```python
from build123d import *

# Parameters (mm, degrees)
CYLINDER003_R     = 3.4
CYLINDER003_DEPTH = 10
CYLINDER004_R     = 1.7
CYLINDER004_DEPTH = 9.6
CYLINDER002_R     = 3.4
CYLINDER002_DEPTH = 10
CYLINDER001_R     = 1.7
CYLINDER001_DEPTH = 9.6
CYLINDER008_R     = 3.4
CYLINDER008_DEPTH = 10
CYLINDER006_R     = 1.7
CYLINDER006_DEPTH = 9.6
CYLINDER005_R     = 3.4
CYLINDER005_DEPTH = 10
CYLINDER007_R     = 1.7
CYLINDER007_DEPTH = 9.6
PAD002_DEPTH      = 2
BOX001_W          = 53
BOX001_H          = 62
BOX001_DEPTH      = 2
FILLET_R          = 3
SKETCH001_W       = 21
SKETCH001_H       = 32
PAD001_DEPTH      = 2


with BuildPart() as grab_screw_head001:
    # Cone002 → Cone002 (revolve)
    with BuildSketch(Plane.XZ):
        Polygon((0, 0), (1.7, 0), (3.4, 3.4), (0, 3.4), align=None)
    revolve(axis=Axis((0, 0, 0), (0, 0, 1)))


with BuildPart() as grab_screw_head_extension001:
    # Cylinder003 → Cylinder003 (new body)
    with BuildSketch(Plane.XY.offset(3.4)):
        Circle(CYLINDER003_R)
    extrude(amount=CYLINDER003_DEPTH)


with BuildPart() as grab_screw001:
    # Cylinder004 → Cylinder004 (new body)
    with BuildSketch(Plane.XY.offset(-9.6)):
        Circle(CYLINDER004_R)
    extrude(amount=CYLINDER004_DEPTH)

    # Fusion002: union grab-screw-head001, grab-screw-head-extension001
    add(grab_screw_head001.part)
    add(grab_screw_head_extension001.part)


with BuildPart() as grab_screw001_1:
    # Fusion002 placement: moved
    add(grab_screw001.part.moved(Location((42, 56, 5))))


with BuildPart() as grab_screw_head:
    # Cone001 → Cone001 (revolve)
    with BuildSketch(Plane.XZ):
        Polygon((0, 0), (1.7, 0), (3.4, 3.4), (0, 3.4), align=None)
    revolve(axis=Axis((0, 0, 0), (0, 0, 1)))


with BuildPart() as grab_screw_head_extension:
    # Cylinder002 → Cylinder002 (new body)
    with BuildSketch(Plane.XY.offset(3.4)):
        Circle(CYLINDER002_R)
    extrude(amount=CYLINDER002_DEPTH)


with BuildPart() as right_screws:
    # Cylinder001 → Cylinder001 (new body)
    with BuildSketch(Plane.XY.offset(-9.6)):
        Circle(CYLINDER001_R)
    extrude(amount=CYLINDER001_DEPTH)

    # Fusion001: union grab-screw-head, grab-screw-head-extension
    add(grab_screw_head.part)
    add(grab_screw_head_extension.part)


with BuildPart() as right_screws_1:
    # Fusion001 placement: moved
    add(right_screws.part.moved(Location((42, 0, 5))))

    # Fusion: union grab-screw001
    add(grab_screw001_1.part)


with BuildPart() as grab_screw_head003:
    # Cone004 → Cone004 (revolve)
    with BuildSketch(Plane.XZ):
        Polygon((0, 0), (1.7, 0), (3.4, 3.4), (0, 3.4), align=None)
    revolve(axis=Axis((0, 0, 0), (0, 0, 1)))


with BuildPart() as grab_screw_head_extension003:
    # Cylinder008 → Cylinder008 (new body)
    with BuildSketch(Plane.XY.offset(3.4)):
        Circle(CYLINDER008_R)
    extrude(amount=CYLINDER008_DEPTH)


with BuildPart() as grab_screw002:
    # Cylinder006 → Cylinder006 (new body)
    with BuildSketch(Plane.XY.offset(-9.6)):
        Circle(CYLINDER006_R)
    extrude(amount=CYLINDER006_DEPTH)

    # Fusion004: union grab-screw-head003, grab-screw-head-extension003
    add(grab_screw_head003.part)
    add(grab_screw_head_extension003.part)


with BuildPart() as grab_screw002_1:
    # Fusion004 placement: moved
    add(grab_screw002.part.moved(Location((42, 56, 5))))


with BuildPart() as grab_screw_head002:
    # Cone003 → Cone003 (revolve)
    with BuildSketch(Plane.XZ):
        Polygon((0, 0), (1.7, 0), (3.4, 3.4), (0, 3.4), align=None)
    revolve(axis=Axis((0, 0, 0), (0, 0, 1)))


with BuildPart() as grab_screw_head_extension002:
    # Cylinder005 → Cylinder005 (new body)
    with BuildSketch(Plane.XY.offset(3.4)):
        Circle(CYLINDER005_R)
    extrude(amount=CYLINDER005_DEPTH)


with BuildPart() as all_screws:
    # Cylinder007 → Cylinder007 (new body)
    with BuildSketch(Plane.XY.offset(-9.6)):
        Circle(CYLINDER007_R)
    extrude(amount=CYLINDER007_DEPTH)

    # Fusion005: union grab-screw-head002, grab-screw-head-extension002
    add(grab_screw_head002.part)
    add(grab_screw_head_extension002.part)


with BuildPart() as all_screws_1:
    # Fusion005 placement: moved
    add(all_screws.part.moved(Location((42, 0, 5))))

    # Fusion003: union grab-screw002
    add(grab_screw002_1.part)


with BuildPart() as all_screws_2:
    # Fusion003 placement: moved
    add(all_screws_1.part.moved(Location((-47, 0, 0))))

    # Fusion006: union right-screws
    add(right_screws_1.part)


with BuildPart() as all_screws_3:
    # Fusion006 placement: moved
    add(all_screws_2.part.moved(Location((0, 0, 12))))


with BuildPart() as compound:
    # Sketch002 → Pad002 (new body)
    with BuildSketch(Plane.XY):
        Polygon((-2.215162, 59.759811), (-2.215162, -3.075415), (38.48941, -3.075415), (45.010048, 28.539799), (36.908657, 47.508923), (23.274607, 59.759811), align=None)
    extrude(amount=PAD002_DEPTH)


with BuildPart() as compound_1:
    # Compound placement: moved
    add(compound.part.moved(Location((0, 0, 20))))


with BuildPart() as fillet_body:
    # Box001 → Box001 (new body)
    with BuildSketch(Plane(origin=(-8, -3, 20), x_dir=(1, 0, 0), z_dir=(0, 0, 1))):
        with Locations((26.5, 31)):
            Rectangle(BOX001_W, BOX001_H)
    extrude(amount=BOX001_DEPTH)

    # Cut: cut Compound
    add(compound_1.part, mode=Mode.SUBTRACT)


with BuildPart() as fillet_body_1:
    # Cut placement: moved
    add(fillet_body.part.moved(Location((0, 0, -22))))

    # Fillet
    fillet_edges = [fillet_body_1.edges().sort_by_distance(p)[0] for p in [
        (-8, -3, -1),
        (-8, 59, -1),
        (45, -3, -1),
        (45, 59, -1),
    ]]
    fillet(fillet_edges, radius=FILLET_R)


with BuildPart() as top_flat:
    # Sketch001 → Pad001 (new body)
    with BuildSketch(Plane.XY):
        Polygon((-2.22, 59.76), (-2.22, -3.08), (38.49, -3.08), (45.010048, 28.539799), (36.908657, 47.508923), (23.274607, 59.76), align=None)
        with Locations((11.28, 33.76)):
            Rectangle(SKETCH001_W, SKETCH001_H, mode=Mode.SUBTRACT)
    extrude(amount=PAD001_DEPTH)


with BuildPart() as top_flat_1:
    # Body001 placement: moved
    add(top_flat.part.moved(Location((0, 0, -2))))

    # Fusion010: union Fillet body
    add(fillet_body_1.part)


with BuildPart() as top_flat_2:
    # Fusion010 placement: moved
    add(top_flat_1.part.moved(Location((0, 0, 19))))

    # Cut001: cut all-screws
    add(all_screws_3.part, mode=Mode.SUBTRACT)


solid = top_flat_2.part
```
Work out the finished part from the listing and answer in its coordinate system (mm). A direction names the side the tool comes from. Give positions to 0.01 mm unless a question says otherwise; leave off trailing zeros. Loops run counter-clockwise (first coordinate to the right, second up) from the corner with the lowest first, then second, coordinate; pieces in that order, holes last. Notation, with made-up numbers: (-1, 60) - (8, 60) arc R34 ccw to (8, 99) - close; hole circle Ø11 at (18, -34). An arc over 180 degrees is marked (long way). Use CSV: the item, a comma, the result in double quotes. Start each with the question number.
(1) Determine the mould class of faces 1 (the face through (-7.14, 58.1, 18.01)), 2 (the face through (18, -3.08, 18)), 3 (the face through (11, 49.76, 18)) for opening direction X: released by +X, released by -X, zero draft, split by the parting line, or undercut.
(2) Find section C-C, the plane z = 18.05. Count the separate pieces of the cut face and the enclosed holes in it, plus the area to 3 significant figures.
(3) Find section A-A, the plane y = 21.5. Determine the outline of the cut face in (x, z), plus the area to 3 significant figures.
(4) Each of these flat-tipped pins is pushed along its axis until it touches: pin 1 (0.6 mm diameter, centred on x = -4, z = 18, fed in from +Y); pin 2 (1 mm diameter, centred on x = -4, z = 17.5, fed in from -Y); pin 3 (0.8 mm diameter, centred on y = 59.5, z = 18.5, fed in from -X). Where does it stop, or does it pass through?
(5) A tool of negligible diameter and unlimited length cuts with its end or side. For faces 4 (the face through (33, 59, 18)), 5 (the face through (-4, 59, 18)), 6 (the face through (0.78, 34, 18)), 7 (the face through (-4, -3, 18)), from which of +Z, -Z, +X, -X, +Y, -Y can it reach the whole face along a straight path? Write none if from no direction.
(6) Find section B-B, the plane x = 5.5. Determine the outline of the cut face in (y, z), plus the area to 3 significant figures.
(7) Find the intervals of material crossed by L1, parallel to X at y = 26.5, z = 18.4; L2, parallel to X at y = 1, z = 18.1; L3, parallel to Y at x = 12.5, z = 18.15, in increasing order.
Results found:
1,face 1,"released by -X"
1,face 2,"zero draft"
1,face 3,"undercut"
2,separate pieces,"1"
2,enclosed holes,"5"
2,area,"2,570 mm^2"
3,outline,"(-8, 17) - (0.78, 17) - (0.78, 19) - (-8, 19) - close; (21.78, 17) - (45, 17) - (45, 19) - (21.78, 19) - close"
3,area,"64.0 mm^2"
4,pin 1,"y = 59"
4,pin 2,"y = -3"
4,pin 3,"x = -2.22"
5,face 4,"+Z, -Z, +X, +Y"
5,face 5,"+Z, -Z, -X, +Y"
5,face 6,"+Z, -Z"
5,face 7,"+Z, -Z, -X, -Y"
6,outline,"(-3.08, 17) - (17.76, 17) - (17.76, 19) - (-3.08, 19) - close; (49.76, 17) - (59.76, 17) - (59.76, 19) - (49.76, 19) - close"
6,area,"61.7 mm^2"
7,L1,"-8 to 0.78, 21.78 to 45"
7,L2,"-8 to -7.02, -2.98 to 39.98, 44.02 to 45"
7,L3,"-3.08 to 17.76, 49.76 to 59.76"
